Input: part model. Units: mm. Frame: model coordinates. Give positions to 0.01 mm unless a question says otherwise; leave off trailing zeros. Order: outer loops, then holes, each group sorted by start corner. A loop starts at its lowest first (then second) coordinate and runs counter-clockwise, first axis right, second up. Notation, with made-up numbers: (87, 76) -> (141, 76) arc R10 ccw to (141, 88) -> close; hole circle Ø9 at (-2, 7). An arc over 180 degrees is marked (long way). Use a Markdown table: item, result. Add a question column.
from build123d import *

# Parameters (mm, degrees)
SKETCH_1_W          = 56
SKETCH_1_H          = 8
EXTRUDE_1_DEPTH     = 38
SKETCH_2_R          = 2.1
CUT_EXTRUDE_1_DEPTH = 69.14690015
SKETCH_3_R          = 1.25
CUT_EXTRUDE_2_DEPTH = 20


with BuildPart() as part:
    # Эскиз1 → Бобышка-Вытянуть1 (new body)
    with BuildSketch(Plane.XY):
        with Locations((28, 4)):
            Rectangle(SKETCH_1_W, SKETCH_1_H)
    extrude(amount=EXTRUDE_1_DEPTH)

    # Эскиз2 → Вырез-Вытянуть1 (cut, through all)
    with BuildSketch(Plane.XY.offset(38)):
        with Locations((4.43, 4)):
            Circle(SKETCH_2_R)
        with Locations((51.57, 4)):
            Circle(SKETCH_2_R)
    extrude(amount=-CUT_EXTRUDE_1_DEPTH, mode=Mode.SUBTRACT)

    # Эскиз3 → Вырез-Вытянуть2 (cut)
    with BuildSketch(Plane(origin=(56, 0, 0), x_dir=(0, 0, -1), z_dir=(1, 0, 0))):
        with Locations((-19, 4)):
            Circle(SKETCH_3_R)
    extrude(amount=-CUT_EXTRUDE_2_DEPTH, mode=Mode.SUBTRACT)


solid = part.part
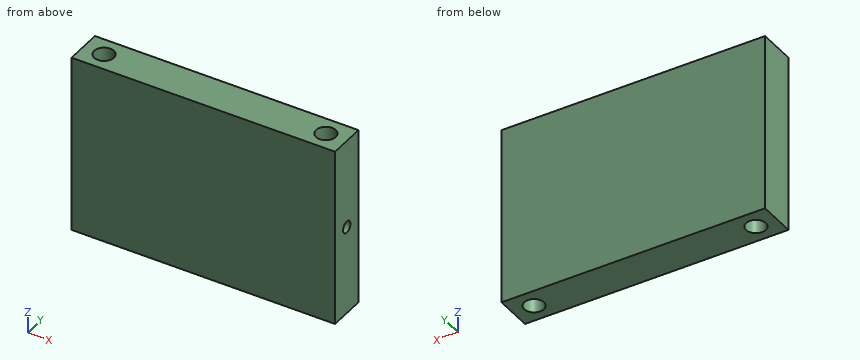
Q1. Section query C-C (z = 19). Return loops of the section in (x, y).
Q2. First-contact query: pin 1 (2 mm diameter, centred on y = 6.5, z = 34, fed in from -X); pin 2 (3.5 mm diameter, centred on x = 51.57, y = 4, fed in from +Z); pin 3 (0.8 mm diameter, centred on y = 4.5, z = 19.5, fed in from +X). Flat tips, straight axial feed; report the tip coordinate or a pass-through.
Q3. Section query A-A (x = 51.57). Return loops of the section in (y, z).
Q4. Ray query, line 1 (Y direction, x = 4.43, z = 28.5); line 2 (Y direction, x = 54.35, z = 19); line 3 (X direction, y = 5.5, z = 13). Return the intervals inside material, ascending.
Q5. Section query B-B (y = 4). Return loops of the section in (x, z).
Q6. Section query D-D (z = 12.5). Return loops of the section in (x, y).
Solution:
| question | item | result |
|---|---|---|
| 1 | outline | (0, 0) -> (56, 0) -> (56, 2.75) -> (53.26, 2.75) arc R2.1 cw to (49.88, 2.75) -> (36, 2.75) -> (36, 5.25) -> (49.88, 5.25) arc R2.1 cw to (53.26, 5.25) -> (56, 5.25) -> (56, 8) -> (0, 8) -> close; hole circle Ø4.2 at (4.43, 4) |
| 2 | pin 1 | stops at x = 0 |
| 2 | pin 2 | passes through |
| 2 | pin 3 | stops at x = 36 |
| 3 | outline | (0, 0) -> (1.9, 0) -> (1.9, 38) -> (0, 38) -> close; (6.1, 0) -> (8, 0) -> (8, 38) -> (6.1, 38) -> close |
| 4 | line 1 | y = 0 to 1.9, 6.1 to 8 |
| 4 | line 2 | y = 0 to 2.75, 5.25 to 8 |
| 4 | line 3 | x = 0 to 2.96, 5.9 to 50.1, 53.04 to 56 |
| 5 | outline | (0, 0) -> (2.33, 0) -> (2.33, 38) -> (0, 38) -> close; (6.53, 0) -> (49.47, 0) -> (49.47, 17.75) -> (36, 17.75) -> (36, 20.25) -> (49.47, 20.25) -> (49.47, 38) -> (6.53, 38) -> close; (53.67, 0) -> (56, 0) -> (56, 17.75) -> (53.67, 17.75) -> close; (53.67, 20.25) -> (56, 20.25) -> (56, 38) -> (53.67, 38) -> close |
| 6 | outline | (0, 0) -> (56, 0) -> (56, 8) -> (0, 8) -> close; hole circle Ø4.2 at (4.43, 4); hole circle Ø4.2 at (51.57, 4) |
